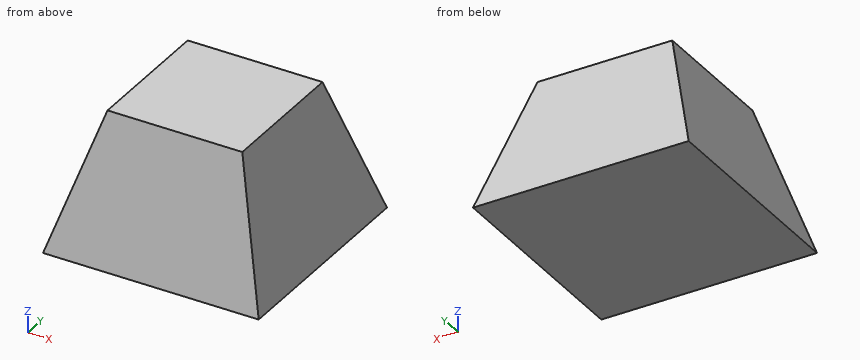
from build123d import *

# Parameters (mm, degrees)
ESBO_O1_W                = 80
ESBO_O1_H                = 80
RESSALTO_EXTRUS_O1_DEPTH = 50
CORTE_EXTRUS_O3_DEPTH    = 103.46950766
CORTE_EXTRUS_O4_DEPTH    = 103.46950766


with BuildPart() as part:
    # Esboço1 → Ressalto-extrusão1 (new body)
    with BuildSketch(Plane.XY):
        Rectangle(ESBO_O1_W, ESBO_O1_H)
    extrude(amount=RESSALTO_EXTRUS_O1_DEPTH)

    # Esboço3 → Corte-extrusão3 (cut, through all)
    with BuildSketch(Plane.ZY.offset(40)):
        Polygon((50, 25), (0, 40), (50, 40), align=None)
        Polygon((50, -25), (0, -40), (50, -40), align=None)
    extrude(amount=-CORTE_EXTRUS_O3_DEPTH, mode=Mode.SUBTRACT)

    # Esboço8 → Corte-extrusão4 (cut, through all)
    with BuildSketch(Plane(origin=(0, -40, 0), x_dir=(-1, 0, 0), z_dir=(0, -1, 0))):
        Polygon((25, -50), (40, 0), (40, -50), align=None)
        Polygon((-25, -50), (-40, -50), (-40, 0), align=None)
    extrude(amount=-CORTE_EXTRUS_O4_DEPTH, mode=Mode.SUBTRACT)


solid = part.part
CAD build for the part. Positions are in the model's coordinates, mm. Give positions to 0.01 mm unless a question says otherwise; leave off trailing zeros. Loops run counter-clockwise (first coordinate to the right, second up) from the corner with the lowest first, then second, coordinate; pieces in that order, holes last. Notation, with made-up numbers: M 41,-24 L 49,-24 A21 cw 49,-17 Z; hole C 7,39 d4. An arc over 180 degrees is marked long. Answer in a Markdown table with one row per item. Add a question column.
Item 1: Band-saw the part on A-A on z = 7.5. Give the cut face in (x, y).
Item 2: Probe probe 1 along Y at (x, z) = (4, 2.5); probe 2 along Y at (x, z) = (17, 30.5); probe 3 along X at (y, z) = (-8, 21.5). List the from-to ranges inside material, lowest first.
Item 3: Drop flat-ended pins along their axis: P1, Ø12, axis at y = 26.5, z = 37.5, coming from the +X side; P2, Ø3, axis at y = 1, z = 43, coming from the +X side; P3, Ø3, axis at y = 26.5, z = 14, coming from the -X side. Give the stop position or say it passes through.
Item 4: Band-saw the part on B-B on x = 5.5. Give the cut face in (y, z), then the cut area to 3 significant figures.
Reply:
| question | item | result |
|---|---|---|
| 1 | outline | M -37.75,-37.75 L 37.75,-37.75 L 37.75,37.75 L -37.75,37.75 Z |
| 2 | probe 1 | y = -39.25 to 39.25 |
| 2 | probe 2 | y = -30.85 to 30.85 |
| 2 | probe 3 | x = -33.55 to 33.55 |
| 3 | P1 | stops at x = 30.55 |
| 3 | P2 | stops at x = 27.55 |
| 3 | P3 | stops at x = -36.25 |
| 4 | outline | M -40,0 L 40,0 L 25,50 L -25,50 Z |
| 4 | area | 3,250 mm^2 |
